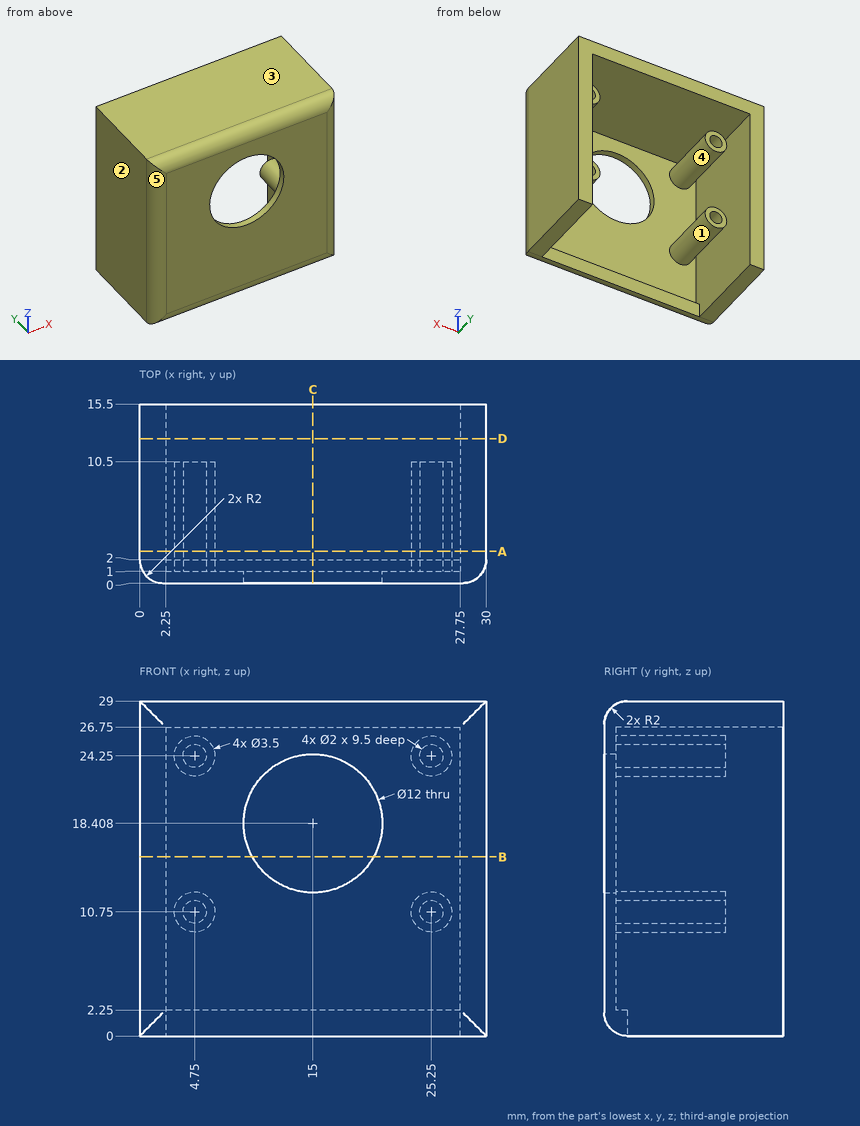
Design review of the part shown in the three views and the two pictorial views. Dimensions are in mm from the part's minimum x, y and z. A direction names the side the tool comes from. Coordinates: 2 decimals unless noted, no trailing zeros. Order: outer loops, then holes, each group sorted by start corner. A loop starts at its lowest first (then second) coordinate and runs counter-clockwise, first axis right, second up.
Item 1: Take a section at B-B, the plane z = 15.5. Write out the cut boundary in (x, y).
Item 2: Take a section at D-D, the plane y = 12.5. Write out the cut boundary in (x, z), then the cut area to 3 significant figures.
Item 3: For line 1 (Z direction, x = 4.75, y = 7.5); line 2 (X direction, y = 3, z = 8.5); line 3 (X direction, y = 8.75, z = 10.75), list the stretches that pass through material, from the lowest coordinate up.
Item 4: Take a section at C-C, the plane x = 15. Write out the cut boundary in (y, z).
Item 5: The part is to be moulded in two halves that separate along Z. For the marked faces 3, 4 and 5, say which applies: pulls with the +Z half, pulls with the -Z half, needs draft (parallel to the pull), parting line crosses it, or undercut.
Item 6: For the marked faces 1 and 2, list the 3-axis set-ups (+Z, -Z, +X, -X, +Y, -Y) from which the entire face can be reached by the end or side of a thin tool; tool diameter is ignored.
Item 7: For pin 1 Ø1.6 at (x, z) = (4.75, 24.25) entering from +Y; pin 2 Ø1.6 at (x, z) = (4.5, 24) entering from +Y; pin 3 Ø7 at (x, y) = (16, 9) entering from -Z, all flat-tipped, find the tip position at first contact; note any pin that passes through.
Item 8: Take a section at A-A, the plane y = 2.75. Count the separate pieces of the cut face and the enclosed holes in it, then the cut area to 3 significant figures.
The answers:
1. outline: (0, 2) arc R2 ccw to (2, 0) - (9.75, 0) - (9.75, 1) - (2.25, 1) - (2.25, 15.5) - (0, 15.5) - close; (20.25, 0) - (28, 0) arc R2 ccw to (30, 2) - (30, 15.5) - (27.75, 15.5) - (27.75, 1) - (20.25, 1) - close
2. outline: (0, 0) - (2.25, 0) - (2.25, 26.75) - (27.75, 26.75) - (27.75, 0) - (30, 0) - (30, 29) - (0, 29) - close
2. area: 188 mm2
3. line 1: z = 9 to 9.75, 11.75 to 12.5, 22.5 to 23.25, 25.25 to 26, 26.75 to 29
3. line 2: x = 0 to 2.25, 27.75 to 30
3. line 3: x = 0 to 2.25, 3 to 3.75, 5.75 to 6.5, 23.5 to 24.25, 26.25 to 27, 27.75 to 30
4. outline: (0, 2) arc R2 ccw to (2, 0) - (2, 2.25) - (1, 2.25) - (1, 12.41) - (0, 12.41) - close; (0, 24.41) - (1, 24.41) - (1, 26.75) - (15.5, 26.75) - (15.5, 29) - (2, 29) arc R2 ccw to (0, 27) - close
5. face 3: pulls with the +Z half
5. face 4: undercut
5. face 5: needs draft
6. face 1: +Y
6. face 2: +Z, -Z, -X, +Y, -Y
7. pin 1: stops at y = 1
7. pin 2: stops at y = 10.5
7. pin 3: stops at z = 26.75
8. separate pieces: 5
8. enclosed holes: 4
8. area: 214 mm2
